Geometry: final body of the model. Coordinates: model frame, mm. A direction names the side the tool comes from. Round coordinates to 2 decimals unless told otherwise and drop trailing zeros. Write each loop counter-clockwise with the first axis right and the second up, starting at its lowest first coordinate (ties: lowest second). Pieces come first, ordered by that corner, then holes. Notation, with made-up numbers: M 49,-2 L 78,-2 A17 cw 78,19 Z; hole C -35,64 d1. An arc over 180 degrees is marked long. Use one line per item in the form item = value. Start each with the question number.
Item 1: Section query C-C (z = -54). Return loops of the section in (x, y), and give its area (3 significant figures).
Item 2: Section query B-B (x = -25). Return loops of the section in (y, z), and give its area (3 significant figures).
Item 3: Ray query, probe 1 along Z at (x, y) = (34, 8); probe 2 along X at (y, z) = (5.5, 54); probe 3 along Y at (x, z) = (11, 48.5). Return the intervals inside material, ascending.
Item 4: Section query A-A (y = 44.5). Return loops of the section in (x, z).
Item 5: Pin query (flat end, axial travel): pin 1 Ø5 at (x, z) = (-20.5, -29) entering from +Y; pin 2 Ø2.5 at (y, z) = (7, 67) entering from -X; pin 3 Ø3.5 at (x, z) = (12.5, 64) entering from +Y. Return the tip coordinate at first contact, or that it passes through.
Item 6: Reachability of faces 4 (the flat face through (-28.815, 10.579, 51.025)), 5 (the flat face through (39.657, 11.4, -37.8)), 6 (the cylindrical face through (-30.892, 8.956, -40.444)), 7 (the flat face through (-6.343, 6, 52)), 8 (the flat face through (-47, 0.8, -64)) from +Z, -Z, +X, -X, +Y, -Y: full face, straight path, thin tool, end or side. Return the list, or none.
Item 7: Section query D-D (y = 26). Return loops of the section in (x, z), and give its area (3 significant figures).
Item 8: Pull-direction query (Z, two-part tool) for faces 1 (the flat face through (32.657, 12, -38)), 2 (the cylindrical face through (56.24, 1.92, 66.34)), 3 (the flat face through (2, 3, -85.944)); classes: pulls with the +Z half, pulls with the -Z half, needs draft (parallel to the pull), parting line crosses it, or undercut.
from build123d import *

# Parameters (mm, degrees)
SKETCH_1_W          = 120
SKETCH_1_H          = 170
EXTRUDE_1_DEPTH     = 4
SKETCH_2_R          = 1.75
CUT_EXTRUDE_1_DEPTH = 107.434596542
SKETCH_3_W          = 7
SKETCH_3_H          = 95
EXTRUDE_2_DEPTH     = 11
SKETCH_4_R          = 2
CUT_EXTRUDE_3_DEPTH = 131.46218131
SKETCH_5_W          = 7
SKETCH_5_H          = 65
EXTRUDE_3_DEPTH     = 46
SKETCH_7_R          = 1.85
SKETCH_7_W          = 42
SKETCH_7_H          = 21
CUT_EXTRUDE_4_DEPTH = 134.77828954
SKETCH_9_W          = 3
SKETCH_9_H          = 65
EXTRUDE_4_DEPTH     = 5
EXTRUDE_5_DEPTH     = 65
SKETCH_13_R         = 4.25
CUT_EXTRUDE_5_DEPTH = 3.2
FILLET_3_R          = 3
FILLET_5_R          = 2
CHAMFER_1_SIZE      = 1
FILLET_6_R          = 2


with BuildPart() as part:
    # 草图1 → 凸台-拉伸1 (new body)
    with BuildSketch(Plane(origin=(0, 0, 0), x_dir=(1, 0, 0), z_dir=(0, 1, 0))):
        with Locations((2.657342657, 0.944055944)):
            Rectangle(SKETCH_1_W, SKETCH_1_H)
    extrude(amount=EXTRUDE_1_DEPTH)

    # 草图2 → 切除-拉伸1 (cut, through all)
    with BuildSketch(Plane(origin=(0, 4, 0), x_dir=(1, 0, 0), z_dir=(0, 1, 0))):
        with Locations(Location((-47.342657343, 65.944055944, 0), (0, 0, 270))):
            Circle(SKETCH_2_R)
        with Locations(Location((-47.342657343, -64.055944056, 0), (0, 0, 90))):
            Circle(SKETCH_2_R)
        with Locations(Location((52.657342657, -64.055944056, 0), (0, 0, 270))):
            Circle(SKETCH_2_R)
        with Locations(Location((52.657342657, 65.944055944, 0), (0, 0, 90))):
            Circle(SKETCH_2_R)
    extrude(amount=-CUT_EXTRUDE_1_DEPTH, mode=Mode.SUBTRACT)

    # 草图3 → 凸台-拉伸2 (add)
    with BuildSketch(Plane(origin=(0, 4, 0), x_dir=(1, 0, 0), z_dir=(0, 1, 0))):
        with Locations((-30.842657343, 38.444055944)):
            Rectangle(SKETCH_3_W, SKETCH_3_H)
        with Locations((36.157342657, 38.444055944)):
            Rectangle(SKETCH_3_W, SKETCH_3_H)
    extrude(amount=EXTRUDE_2_DEPTH)

    # 草图4 → 切除-拉伸3 (cut, through all)
    with BuildSketch(Plane.ZY.offset(34.342657343)):
        with Locations((-78.444055944, 9)):
            Circle(SKETCH_4_R)
        with BuildLine():
            Line((-38.444055944, 11), (1.555944056, 11))
            ThreePointArc((1.555944056, 11), (3.555944056, 9), (1.555944056, 7))
            Line((1.555944056, 7), (-38.444055944, 7))
            ThreePointArc((-38.444055944, 7), (-40.444055944, 9), (-38.444055944, 11))
        make_face()
    extrude(amount=-CUT_EXTRUDE_3_DEPTH, mode=Mode.SUBTRACT)

    # 草图5 → 凸台-拉伸3 (add)
    with BuildSketch(Plane(origin=(0, 4, 0), x_dir=(1, 0, 0), z_dir=(0, 1, 0))):
        with Locations((-23.342657343, -51.555944056)):
            Rectangle(SKETCH_5_W, SKETCH_5_H)
    extrude(amount=EXTRUDE_3_DEPTH)

    # 草图7 → 切除-拉伸4 (cut, through all)
    with BuildSketch(Plane.ZY.offset(26.842657343)):
        with Locations((27.305944056, 34.5)):
            Circle(SKETCH_7_R)
        with Locations((27.305944056, 44.5)):
            Circle(SKETCH_7_R)
        with Locations((75.805944056, 44.5)):
            Circle(SKETCH_7_R)
        with Locations((75.805944056, 34.5)):
            Circle(SKETCH_7_R)
        with Locations((51.555944056, 39.5)):
            Rectangle(SKETCH_7_W, SKETCH_7_H)
    extrude(amount=-CUT_EXTRUDE_4_DEPTH, mode=Mode.SUBTRACT)

    # 草图9 → 凸台-拉伸4 (add)
    with BuildSketch(Plane(origin=(0, 4, 0), x_dir=(1, 0, 0), z_dir=(0, 1, 0))):
        with Locations((-7.842657343, -51.555944056)):
            Rectangle(SKETCH_9_W, SKETCH_9_H)
        with Locations((12.157342657, -51.555944056)):
            Rectangle(SKETCH_9_W, SKETCH_9_H)
    extrude(amount=EXTRUDE_4_DEPTH)

    # 草图11 → 凸台-拉伸5 (add)
    with BuildSketch(Plane(origin=(-26.842657343, 4, 84.055944056), x_dir=(1, 0, 0), z_dir=(0, 0, 1))):
        Polygon((0, 12.976482023), (-4, 0), (0, 0), align=None)
        Polygon((7, 0), (11, 0), (7, 12.976482023), align=None)
    extrude(amount=-EXTRUDE_5_DEPTH)

    # 草图13 → 切除-拉伸5 (cut)
    with BuildSketch(Plane(origin=(0, 4, 0), x_dir=(1, 0, 0), z_dir=(0, 1, 0))):
        with Locations(Location((-47.342657343, 65.944055944, 0), (0, 0, 270))):
            Circle(SKETCH_13_R)
        with Locations(Location((52.657342657, 65.944055944, 0), (0, 0, 90))):
            Circle(SKETCH_13_R)
        with Locations(Location((52.657342657, -64.055944056, 0), (0, 0, 270))):
            Circle(SKETCH_13_R)
        with Locations(Location((-47.342657343, -64.055944056, 0), (0, 0, 90))):
            Circle(SKETCH_13_R)
    extrude(amount=-CUT_EXTRUDE_5_DEPTH, mode=Mode.SUBTRACT)

    # 圆角3
    fillet_3_edges = [part.edges().sort_by_distance(p)[0] for p in [
        (-57.342657343, 4, -0.944055944),
        (62.657342657, 4, -0.944055944),
    ]]
    fillet(fillet_3_edges, radius=FILLET_3_R)

    # 圆角5
    fillet_5_edges = [part.edges().sort_by_distance(p)[0] for p in [
        (-9.342657343, 4, 51.555944056),
        (13.657342657, 4, 51.555944056),
    ]]
    fillet(fillet_5_edges, radius=FILLET_5_R)

    # 倒角1
    chamfer_1_edges = [part.edges().sort_by_distance(p)[0] for p in [
        (-47.342657343, 4, 68.305944056),
        (52.657342657, 4, 59.805944056),
        (52.657342657, 4, -61.694055944),
        (-47.342657343, 4, -70.194055944),
    ]]
    chamfer(chamfer_1_edges, length=CHAMFER_1_SIZE)

    # 圆角6
    fillet_6_edges = [part.edges().sort_by_distance(p)[0] for p in [
        (-23.342657343, 4, 19.055944056),
        (-23.342657343, 50, 84.055944056),
        (-23.342657343, 50, 19.055944056),
        (-23.342657343, 50, 72.555944056),
        (-23.342657343, 50, 30.555944056),
        (-7.842657343, 9, 84.055944056),
        (-7.842657343, 9, 19.055944056),
        (12.157342657, 9, 84.055944056),
        (12.157342657, 9, 19.055944056),
        (-34.342657343, 4, -38.444055944),
        (-30.842657343, 15, 9.055944056),
        (-30.842657343, 15, -85.944055944),
        (36.157342657, 15, 9.055944056),
        (36.157342657, 15, -85.944055944),
        (39.657342657, 4, -38.444055944),
    ]]
    fillet(fillet_6_edges, radius=FILLET_6_R)


solid = part.part
Working result:
q1.outline = M -57.34,0 L 62.66,0 L 62.66,1 A3 ccw 59.66,4 L 41.66,4 A2 cw 39.66,6 L 39.66,15 L 32.66,15 L 32.66,4 L -27.34,4 L -27.34,15 L -34.34,15 L -34.34,6 A2 cw -36.34,4 L -54.34,4 A3 ccw -57.34,1 Z
q1.area = 632 mm²
q2.outline = M 0,-85.94 L 4,-85.94 L 4,17.06 A2 cw 6,19.06 L 48,19.06 A2 ccw 50,21.06 L 50,28.56 A2 ccw 48,30.56 L 29,30.56 L 29,72.56 L 48,72.56 A2 ccw 50,74.56 L 50,82.06 A2 ccw 48,84.06 L 0,84.06 Z; hole C 34.5,27.31 d3.7; hole C 34.5,75.81 d3.7; hole C 44.5,27.31 d3.7; hole C 44.5,75.81 d3.7
q2.area = 2,740 mm²
q3.probe_1 = -85.94 to -80.18, -76.71 to -40.18, 3.29 to 9.06
q3.probe_2 = -30.38 to -16.31, -9.41 to -6.34, 10.66 to 13.72
q3.probe_3 = 0 to 9
q4.outline = M -26.84,19.06 L -19.84,19.06 L -19.84,25.46 L -26.84,25.46 Z; M -26.84,29.16 L -19.84,29.16 L -19.84,30.56 L -26.84,30.56 Z; M -26.84,72.56 L -19.84,72.56 L -19.84,73.96 L -26.84,73.96 Z; M -26.84,77.66 L -19.84,77.66 L -19.84,84.06 L -26.84,84.06 Z
q5.pin_1 = 4
q5.pin_2 = -30.3
q5.pin_3 = 9
q6.face_4 = +Z, -X, +Y
q6.face_5 = +Z, -Z, +X, +Y
q6.face_6 = +X, -X
q6.face_7 = +Z, -Z, +Y
q6.face_8 = +Y
q7.outline = M -26.84,19.06 L -19.84,19.06 L -19.84,84.06 L -26.84,84.06 Z
q7.area = 455 mm²
q8.face_1 = needs draft
q8.face_2 = undercut
q8.face_3 = pulls with the -Z half
